CAD build for the part. Positions are in the model's coordinates, mm. A direction names the side the tool comes from. Give positions to 0.01 mm unless a question says otherwise; leave off trailing zeros. Order: outer loops, then holes, each group sorted by start corner. A loop starts at its lowest first (then second) coordinate and runs counter-clockwise, first axis right, second up.
from build123d import *
from build123d.topology import SkipClean

# Parameters (mm, degrees)
SKETCH2_R                = 7.62
BOSS_EXTRUDE1_DEPTH      = 50.8
SKETCH2_R_2              = 7.619999999999999
BOSS_EXTRUDE1_2_DEPTH    = 50.8
SKETCH4_W                = 15.239999999999998
SKETCH4_H                = 15.239999999999998
BOSS_EXTRUDE3_DEPTH      = 15.239999999999998
SKETCH6_W                = 15.240000000000016
SKETCH6_H                = 15.239999999999998
BOSS_EXTRUDE4_DEPTH      = 25.4
SKETCH7_R                = 7.619999999999997
BOSS_EXTRUDE6_DEPTH      = 38.1
CUT_EXTRUDE1_DEPTH       = 86.10600000000002
CUT_EXTRUDE2_START       = -86.10600000000002
CUT_EXTRUDE2_DEPTH       = 86.10600000000002
BOSS_EXTRUDE7_DEPTH      = 50.8
BOSS_EXTRUDE7_DEPTH_BACK = 15.239999999999998
SKETCH10_W               = 15.239999999999998
SKETCH10_H               = 15.240000000000016
CUT_EXTRUDE6_DEPTH       = 92.45600000000002


with BuildPart() as part:
    # Sketch2 → Boss-Extrude1 (new body)
    with BuildSketch(Plane.XY):
        Circle(SKETCH2_R)
    extrude(amount=BOSS_EXTRUDE1_DEPTH)

    # Sketch4 → Boss-Extrude3 (add)
    with BuildSketch(Plane.XY.offset(50.8)):
        Rectangle(SKETCH4_W, SKETCH4_H)
    extrude(amount=BOSS_EXTRUDE3_DEPTH)

    # Sketch6 → Boss-Extrude4 (add)
    with BuildSketch(Plane(origin=(7.619999999999999, 0, 0), x_dir=(0, 0, -1), z_dir=(1, 0, 0))):
        with Locations((-58.42, 0)):
            Rectangle(SKETCH6_W, SKETCH6_H)
    extrude(amount=BOSS_EXTRUDE4_DEPTH)

    # Sketch7 → Boss-Extrude6 (add)
    with BuildSketch(Plane.XY.offset(66.04)):
        with Locations((25.400000000000002, 0)):
            Circle(SKETCH7_R)
    extrude(amount=BOSS_EXTRUDE6_DEPTH)

    # Sketch8 → Cut-Extrude1 (cut)
    with BuildSketch(Plane(origin=(0, 0, 0), x_dir=(-1, 0, 0), z_dir=(0, 0, -1))):
        with BuildLine():
            Line((7.619999999999999, 0), (7.619999999999999, 7.619999999999999))
            Line((7.619999999999999, 7.619999999999999), (3.2596e-13, 7.619999999999999))
            ThreePointArc((3.2702e-13, 7.62), (5.388153672641607, 5.388153672641376), (7.62, 0))
        make_face()
        with BuildLine():
            Line((7.619999999999999, -7.619999999999997), (7.619999999999999, 0))
            ThreePointArc((7.62, -1.87e-15), (5.3881536742144505, -5.388153671068534), (4.44899204e-09, -7.62))
            Line((4.44899229e-09, -7.619999999999997), (7.619999999999999, -7.619999999999997))
        make_face()
    extrude(amount=-CUT_EXTRUDE1_DEPTH, mode=Mode.SUBTRACT)

    # Sketch9 → Cut-Extrude2 (cut)
    with BuildSketch(Plane.XY.offset(104.14000000000001).offset(CUT_EXTRUDE2_START)):
        with BuildLine():
            Line((33.02, 0), (33.02, 7.619999999999999))
            Line((33.02, 7.619999999999999), (25.40000000000031, 7.619999999999999))
            ThreePointArc((25.40000000000031, 7.619999999999997), (30.788153672641602, 5.388153672641381), (33.019999999999996, 0))
        make_face()
        with BuildLine():
            Line((33.02, -7.619999999999997), (33.02, 0))
            ThreePointArc((33.019999999999996, -1.87e-15), (30.788153672641606, -5.388153672641376), (25.400000000000325, -7.619999999999997))
            Line((25.400000000000325, -7.619999999999997), (33.02, -7.619999999999997))
        make_face()
    extrude(amount=CUT_EXTRUDE2_DEPTH, mode=Mode.SUBTRACT)



with BuildPart() as body_2:
    # Sketch2 → Boss-Extrude1 2 (new body)
    with BuildSketch(Plane.XY):
        with Locations((6.22e-15, -50.8)):
            Circle(SKETCH2_R_2)
    extrude(amount=BOSS_EXTRUDE1_2_DEPTH)


with BuildPart() as part_1:
    add(part.part)

    add(body_2.part)  # Boss-Extrude7 merges body 2
    # Sketch10 → Boss-Extrude7 (add, two sides: drawn at the far end of the back side and taken through both)
    with BuildSketch(Plane.XZ.offset(7.619999999999999).offset(-BOSS_EXTRUDE7_DEPTH_BACK)):
        with Locations((0, 58.42)):
            Rectangle(SKETCH10_W, SKETCH10_H)
    extrude(amount=BOSS_EXTRUDE7_DEPTH + BOSS_EXTRUDE7_DEPTH_BACK)

    # Sketch13 → Cut-Extrude6 (cut)
    with SkipClean():  # the faces are left unmerged after this step: merging them gives an invalid solid
        with BuildSketch(Plane(origin=(0, 0, 0), x_dir=(-1, 0, 0), z_dir=(0, 0, -1))):
            with BuildLine():
                Line((7.619999999999999, 0), (7.619999999999999, 7.619999999999999))
                Line((7.619999999999999, 7.619999999999999), (3.2685e-13, 7.619999999999999))
                ThreePointArc((3.2702e-13, 7.62), (5.388153672641607, 5.388153672641376), (7.62, 0))
            make_face()
            with BuildLine():
                Line((3.895929446e-08, -58.42), (7.619999999999999, -58.42))
                Line((7.619999999999999, -58.42), (7.619999999999999, -50.8))
                ThreePointArc((7.619999999999991, -50.8), (5.388153686415675, -56.18815365886729), (3.895929121e-08, -58.419999999999995))
            make_face()
            with BuildLine():
                Line((-7.619999999999999, -58.42), (3.895929446e-08, -58.42))
                ThreePointArc((3.895929121e-08, -58.419999999999995), (-5.388153658867306, -56.18815368641568), (-7.620000000000004, -50.8))
                Line((-7.619999999999998, -50.8), (-7.619999999999998, -58.42))
            make_face()
        extrude(amount=-CUT_EXTRUDE6_DEPTH, mode=Mode.SUBTRACT)


solid = part_1.part
1. Saw through at A-A on z = 21. Give the cut face in (x, y).
2. 3-axis set-ups, long thin cutter, end or side, ignore diameter. For faces 1 (the flat face through (7.62, -29, 58)), 2 (the cylindrical face through (32.47, 2.84, 77.1)), 3 (the flat face through (0, 0, 0)): which of +Z, -Z, +X, -X, +Y, -Y reach the whole face in a straight line?
3. Wall check: line 1 (X direction, y = -0.5, z = 77); line 2 (X direction, y = -33, z = 63.5); line 3 (Z direction, x = 2.5, y = -28). Give the ranges that are in metal, low to high.
4. Saw through at B-B on z = 63.5. Give the cut face in (x, y).
5. Pin check, flat tips, straight feed: P1, Ø8, axis at y = -24, z = 46, coming from the +X side; P2, Ø1.5, axis at x = 7, z = 50, coming from the +Y side; P3, Ø17, axis at x = 19.5, z = 60, coming from the -Y side; P4, Ø7.5, axis at y = -30, z = 60.5, coming from the +X side. Stop position of each tip, or through.
6. Saw through at D-D on y = -6.5. Give the cut face in (x, z).
7. Saw through at C-C on x = 2.5. Give the cut face in (y, z), plus the area to 3 significant figures.
8. Mould opens along Y. For faces 4 (the flat face through (13, 7.62, 59)), 5 (the flat face through (25, 0, 104.14)), 6 (the flat face through (16, -7.62, 59)), 7 (the flat face through (3, -15, 50.8)) say: released by +Y, released by -Y, zero draft, split by the parting line, or undercut.
Reported:
1. outline: circle Ø15.24 at (0, -50.8); circle Ø15.24 at (0, 0)
2. face 1: +Z, -Z, +X, -Y
2. face 2: +Z
2. face 3: -Z, +X, -X, +Y, -Y
3. line 1: x = 17.8 to 33
3. line 2: x = -7.62 to 7.62
3. line 3: z = 50.8 to 66.04
4. outline: (-7.62, -50.8) arc R7.62 ccw to (7.62, -50.8) - (7.62, -7.62) - (25.4, -7.62) arc R7.62 ccw to (25.4, 7.62) - (0, 7.62) arc R7.62 ccw to (-7.62, 0) - close
5. P1: passes through
5. P2: stops at y = 4.36
5. P3: stops at y = -7.62
5. P4: stops at x = 7.62
6. outline: (-7.62, 50.8) - (-3.98, 50.8) - (-3.98, 0) - (3.98, 0) - (3.98, 50.8) - (29.38, 50.8) - (29.38, 104.14) - (21.42, 104.14) - (21.42, 66.04) - (-7.62, 66.04) - close
7. outline: (-58, 0) - (-43.6, 0) - (-43.6, 50.8) - (-7.2, 50.8) - (-7.2, 0) - (7.2, 0) - (7.2, 50.8) - (7.62, 50.8) - (7.62, 66.04) - (-58, 66.04) - close
7. area: 2,460 mm2
8. face 4: released by +Y
8. face 5: zero draft
8. face 6: released by -Y
8. face 7: undercut
